Verification items for the finished model (mm, model axes). A direction names the side the tool comes from. Round coordinates to 2 decimals unless told otherwise and drop trailing zeros. Loops run counter-clockwise (first coordinate to the right, second up) from the corner with the lowest first, then second, coordinate; pieces in that order, holes last. Notation, with made-up numbers: (78, -31.75) - (112, -31.75) arc R16 ccw to (112, -23.75) - close; hole circle Ø4 at (44, 89.5). An arc over 180 degrees is marked (long way). Use CSV: the item, a comma, the result in double quotes.
```python
from build123d import *

# Parameters (mm, degrees)
SKETCH1_R           = 7
SKETCH1_R_2         = 1
BOSS_EXTRUDE1_DEPTH = 4
CUT_EXTRUDE2_DEPTH  = 5
CIRPATTERN2_COUNT   = 12
SKETCH11_R          = 4.5
BOSS_EXTRUDE2_DEPTH = 11
CUT_EXTRUDE3_START  = 11
CUT_EXTRUDE3_DEPTH  = 2
CUT_EXTRUDE4_DEPTH  = 12


with BuildPart() as part:
    # Sketch1 → Boss-Extrude1 (new body)
    with BuildSketch(Plane.XY):
        Circle(SKETCH1_R)
        Circle(SKETCH1_R_2, mode=Mode.SUBTRACT)
    extrude(amount=BOSS_EXTRUDE1_DEPTH)

    # Sketch4 → Cut-Extrude2 (cut, through all)
    with BuildSketch(Plane.XY):
        with BuildLine():
            ThreePointArc((-0.50015724, 4.97492138), (0, 5), (0.50015724, 4.97492138))
            ThreePointArc((0.50015724, 4.97492138), (1.158572372, 6.483432479), (2.72550834, 6.98724583))
            ThreePointArc((2.72550834, 6.98724583), (0, 7.5), (-2.72550834, 6.98724583))
            ThreePointArc((-2.72550834, 6.98724583), (-1.167899531, 6.491813775), (-0.5, 5))
            ThreePointArc((-0.5, 5), (-0.500039311, 4.987460443), (-0.50015724, 4.97492138))
        make_face()
    cut_extrude2 = extrude(amount=CUT_EXTRUDE2_DEPTH, mode=Mode.SUBTRACT)

    # CirPattern2: Cut-Extrude2 ×12 about axis
    cirpattern2_axis = Axis((0, 0, 0), (0, 0, 1))
    for i in range(1, CIRPATTERN2_COUNT):
        add(cut_extrude2.rotate(cirpattern2_axis, i * 360 / CIRPATTERN2_COUNT), mode=Mode.SUBTRACT)

    # Sketch11 → Boss-Extrude2 (add)
    with BuildSketch(Plane.XY):
        Circle(SKETCH11_R)
    extrude(amount=BOSS_EXTRUDE2_DEPTH)

    # Sketch12 → Cut-Extrude3 (cut)
    with BuildSketch(Plane.XY.offset(CUT_EXTRUDE3_START)):
        Polygon((3.290896534, 0), (1.645448267, 2.85), (-1.645448267, 2.85), (-3.290896534, 0), (-1.645448267, -2.85), (1.645448267, -2.85), align=None)
    extrude(amount=-CUT_EXTRUDE3_DEPTH, mode=Mode.SUBTRACT)

    # Sketch13 → Cut-Extrude4 (cut, through all)
    with BuildSketch(Plane.XY):
        with BuildLine():
            Line((1.6, 0.95), (-1.6, 0.95))
            ThreePointArc((-1.6, 0.95), (0, -1.860779407), (1.6, 0.95))
        make_face()
    extrude(amount=CUT_EXTRUDE4_DEPTH, mode=Mode.SUBTRACT)


solid = part.part
```
1) Cross-section at D-D, the plane x = 3.75. Record the cut outline in (y, z), then the cut area to 3 significant figures.
Returned:
outline,"(-4.86, 0) - (4.86, 0) - (4.86, 4) - (2.49, 4) - (2.49, 11) - (-2.49, 11) - (-2.49, 4) - (-4.86, 4) - close"
area,"73.7 mm²"
2) Cross-section at C-C, the plane z = 7. Record the cut outline in (x, y), then the cut area to 3 significant figures.
Returned:
outline,"circle Ø9 at (0, 0); hole (-1.6, 0.95) arc R1.86 ccw (long way) to (1.6, 0.95) - close"
area,"54.8 mm²"
3) Mould release check, pull along X, two halves, no side actions. Record for faces 1 (the face through (-1, 5, 4)), 2 (the face through (0, 1.3, 9)), 3 (the face through (-6.081, -0.817, 1.972)): +X half, -X half, draft (parallel to the pull), parting line (faces both ways), or undercut.
Returned:
face 1,"draft"
face 2,"undercut"
face 3,"-X half"
4) Access from +Z, -Z, +X, -X, +Y, -Y to the whole of each face (thin tool, end or side, straight path). Record for faces 4 (the face through (-4.327, -2.506, 1.972)), 5 (the face through (2.48, 1.405, 10.014)), 6 (the face through (3.75, -4.86, 1.97)).
Returned:
face 4,"+Z, -Z"
face 5,"+Z"
face 6,"+Z, -Z, -Y"
5) Cross-section at A-A, the plane x = 0. Record the cut outline in (y, z).
Returned:
outline,"(-5, 0) - (-1.86, 0) - (-1.86, 9) - (-2.85, 9) - (-2.85, 11) - (-4.5, 11) - (-4.5, 4) - (-5, 4) - close; (0.95, 0) - (5, 0) - (5, 4) - (4.5, 4) - (4.5, 11) - (2.85, 11) - (2.85, 9) - (0.95, 9) - close"
6) Cross-section at B-B, the plane y = 5.5. Record the cut outline in (x, z).
Returned:
outline,"(-2.33, 0) - (-0.56, 0) - (-0.56, 4) - (-2.33, 4) - close; (0.56, 0) - (2.33, 0) - (2.33, 4) - (0.56, 4) - close"
7) Thickness scan on probe 1 along X at (y, z) = (0, 7); probe 2 along Y at (x, z) = (0, 2.5); probe 3 along X at (y, z) = (0.5, 7.75). Record the ranges inside material, lowest first. Write a range as [from, to].
Returned:
probe 1,"x = [-4.5, -1.86], [1.86, 4.5]"
probe 2,"y = [-5, -1.86], [0.95, 5]"
probe 3,"x = [-4.47, -1.79], [1.79, 4.47]"
8) Gauge pin test, flat ends, axial feed: pin 1 Ø2 at (x, z) = (0, 10) entering from +Y; pin 2 Ø1.5 at (x, z) = (-4.5, 4.5) entering from +Y; pin 3 Ø3 at (x, y) = (-1, 0) entering from +Z. Record the tip position at first contact, or that the pin passes through.
Returned:
pin 1,"stops at y = 4.5"
pin 2,"stops at y = 5.08"
pin 3,"stops at z = 9"
